Source: CAD feature listing. Evaluate the final solid. Frame: model axes, mm. A direction names the side the tool comes from. Round coordinates to 2 decimals unless told otherwise and drop trailing zeros. Loops run counter-clockwise (first coordinate to the right, second up) from the corner with the lowest first, then second, coordinate; pieces in that order, holes last. Notation, with made-up numbers: M 62,-30 L 111,-30 A20 ccw 111,-10 Z; hole C 21,38 d9. An arc over 180 degrees is marked long. Write each question's results on one line, items separated by ' | '. Start each with the question number.
1. Section B-B on z = -5. Output: boundary loops of the cut face in (x, y), and give its area (3 significant figures).
2. Draft query along Z for faces 1 (the flat face through (20, 3, -30)), 2 (the flat face through (0, 3, -15)), 3 (the cylindrical face through (36.464, 3.042, -4.675)). Return one class per face: released by +Z, released by -Z, zero draft, split by the parting line, or undercut.
3. Section A-A on x = 16. Output: boundary loops of the cut face in (y, z).
4. Set-up query: faces 4 (the flat face through (15.5, 5, -15)), 5 (the flat face through (25.5, 5.4, -15)), 6 (the flat face through (11.22, 1.53, -14.87)). Return all of +Z, -Z, +X, -X, +Y, -Y with unobstructed straight access to the full face (end or side cutting, diameter ignored); none if empty.
5. Contact query for flat-ended pins moving along their axis: pin 1 Ø5 at (x, z) = (35, -25) entering from +Y; pin 2 Ø2 at (x, z) = (16, -24) entering from +Y. Output: stop coordinate, or through.
6. Ray query, line 1 (X direction, y = 3.85, z = -25); line 2 (Z direction, x = 21, y = 5.75); line 3 (X direction, y = 1.55, z = -25). Return the intervals inside material, ascending.
7. Section C-C on x = 35. Output: boundary loops of the cut face in (y, z).
8. Section D-D on y = 0.5. Output: boundary loops of the cut face in (x, z).
from build123d import *
from OCP.BRepFilletAPI import BRepFilletAPI_MakeChamfer

# Parameters (mm, degrees)
SKETCH1_W           = 40
SKETCH1_H           = 30
BOSS_EXTRUDE1_DEPTH = 6
SKETCH2_R           = 1.5
CUT_EXTRUDE1_DEPTH  = 6
FILLET1_R           = 4
SKETCH3_W           = 21
SKETCH3_H           = 21
CUT_EXTRUDE2_DEPTH  = 4
SKETCH6_W           = 9
SKETCH6_H           = 5
CUT_EXTRUDE3_DEPTH  = 2
SKETCH7_W           = 11
SKETCH7_H           = 7
SKETCH7_W_2         = 9
SKETCH7_H_2         = 5
BOSS_EXTRUDE2_DEPTH = 4
CHAMFER1_SIZE       = 4
CHAMFER1_SIZE2      = 6.92820323
CHAMFER2_SIZE       = 2.886751346
CHAMFER2_SIZE_2     = 5


with BuildPart() as part:
    # Sketch1 → Boss-Extrude1 (new body)
    with BuildSketch(Plane(origin=(0, 0, 0), x_dir=(1, 0, 0), z_dir=(0, 1, 0))):
        with Locations((20, 15)):
            Rectangle(SKETCH1_W, SKETCH1_H)
    extrude(amount=BOSS_EXTRUDE1_DEPTH)

    # Sketch2 → Cut-Extrude1 (cut)
    with BuildSketch(Plane(origin=(0, 6, 0), x_dir=(1, 0, 0), z_dir=(0, 1, 0))):
        with Locations(Location((5, 5, 0), (0, 0, 270))):
            Circle(SKETCH2_R)
        with Locations(Location((5, 25, 0), (0, 0, 90))):
            Circle(SKETCH2_R)
        with Locations(Location((35, 5, 0), (0, 0, 90))):
            Circle(SKETCH2_R)
        with Locations(Location((35, 25, 0), (0, 0, 270))):
            Circle(SKETCH2_R)
    extrude(amount=-CUT_EXTRUDE1_DEPTH, mode=Mode.SUBTRACT)

    # Fillet1
    fillet1_edges = [part.edges().sort_by_distance(p)[0] for p in [
        (0, 3, -30),
        (40, 3, -30),
        (40, 3, 0),
        (0, 3, 0),
    ]]
    fillet(fillet1_edges, radius=FILLET1_R)

    # Sketch3 → Cut-Extrude2 (cut)
    with BuildSketch(Plane(origin=(0, 6, 0), x_dir=(1, 0, 0), z_dir=(0, 1, 0))):
        with Locations((20, 15)):
            Rectangle(SKETCH3_W, SKETCH3_H)
    extrude(amount=-CUT_EXTRUDE2_DEPTH, mode=Mode.SUBTRACT)

    # Sketch6 → Cut-Extrude3 (cut)
    with BuildSketch(Plane(origin=(0, 2, 0), x_dir=(1, 0, 0), z_dir=(0, 1, 0))):
        with Locations((20, 15)):
            Rectangle(SKETCH6_W, SKETCH6_H)
    extrude(amount=-CUT_EXTRUDE3_DEPTH, mode=Mode.SUBTRACT)

    # Sketch7 → Boss-Extrude2 (add)
    with BuildSketch(Plane(origin=(0, 2, 0), x_dir=(1, 0, 0), z_dir=(0, 1, 0))):
        with Locations((20, 15)):
            Rectangle(SKETCH7_W, SKETCH7_H)
        with Locations((20, 15)):
            Rectangle(SKETCH7_W_2, SKETCH7_H_2, mode=Mode.SUBTRACT)
    extrude(amount=BOSS_EXTRUDE2_DEPTH)

    # Chamfer1: one chamfer whose edges measure the first distance from different faces: ONE call of the kernel's chamfer builder (chamfer() names one face for all edges)
    chamfer1_edges_1 = [part.edges().sort_by_distance(p)[0] for p in [
        (20, 0, -12.5),
    ]]
    chamfer1_side_1 = [part.faces().sort_by_distance(p)[0] for p in [
        (20, 3, -12.5),
    ]]
    chamfer1_edges_2 = [part.edges().sort_by_distance(p)[0] for p in [
        (24.5, 0, -15),
    ]]
    chamfer1_side_2 = [part.faces().sort_by_distance(p)[0] for p in [
        (24.5, 3, -15),
    ]]
    chamfer1_edges_3 = [part.edges().sort_by_distance(p)[0] for p in [
        (20, 0, -17.5),
    ]]
    chamfer1_side_3 = [part.faces().sort_by_distance(p)[0] for p in [
        (20, 3, -17.5),
    ]]
    chamfer1_edges_4 = [part.edges().sort_by_distance(p)[0] for p in [
        (15.5, 0, -15),
    ]]
    chamfer1_side_4 = [part.faces().sort_by_distance(p)[0] for p in [
        (15.5, 3, -15),
    ]]
    chamfer1 = BRepFilletAPI_MakeChamfer(part.part.solid().wrapped)
    for e in chamfer1_edges_1:
        chamfer1.Add(CHAMFER1_SIZE, CHAMFER1_SIZE2, e.wrapped, chamfer1_side_1[0].wrapped)  # the first distance lies on this face
    for e in chamfer1_edges_2:
        chamfer1.Add(CHAMFER1_SIZE, CHAMFER1_SIZE2, e.wrapped, chamfer1_side_2[0].wrapped)  # the first distance lies on this face
    for e in chamfer1_edges_3:
        chamfer1.Add(CHAMFER1_SIZE, CHAMFER1_SIZE2, e.wrapped, chamfer1_side_3[0].wrapped)  # the first distance lies on this face
    for e in chamfer1_edges_4:
        chamfer1.Add(CHAMFER1_SIZE, CHAMFER1_SIZE2, e.wrapped, chamfer1_side_4[0].wrapped)  # the first distance lies on this face
    add(Compound.cast(chamfer1.Shape()), mode=Mode.REPLACE)

    # Chamfer2
    # the kernel refuses this chamfer: 5, 2.886751346 mm, written as the material it adds along each edge
    with BuildSketch(Plane(origin=(14.5, 2, -31.435428773), x_dir=(0, 1, 0), z_dir=(0, 0, 1))) as chamfer2_piece_1_section:
        Polygon((CHAMFER2_SIZE, 0), (0, CHAMFER2_SIZE_2), (0, 0), align=None)
    chamfer2_piece_1 = extrude(amount=32.870857546, mode=Mode.PRIVATE)
    chamfer2_piece_1 = split(chamfer2_piece_1, bisect_by=Plane(origin=(13.883974596, 3.066987298, -31.435428773), z_dir=(-0.499999999999998, 0.8660254037844398, 0)), keep=Keep.TOP, mode=Mode.PRIVATE)
    chamfer2_piece_1 = split(chamfer2_piece_1, bisect_by=Plane(origin=(14.5, -1.436141454, -29.45157158), z_dir=(0, -0.8660254037844382, 0.500000000000001)), keep=Keep.TOP, mode=Mode.PRIVATE)
    chamfer2_piece_1 = split(chamfer2_piece_1, bisect_by=Plane(origin=(14.5, 12.797357386, -25.20157158), z_dir=(0, -0.8660254037844382, -0.500000000000001)), keep=Keep.TOP, mode=Mode.PRIVATE)
    with BuildSketch(Plane(origin=(14.5, 2, -31.435428773), x_dir=(0, 1, 0), z_dir=(0, 0, 1))) as chamfer2_piece_2_section:
        Polygon((CHAMFER2_SIZE, 0), (0, CHAMFER2_SIZE_2), (0, 0), align=None)
    chamfer2_piece_2 = extrude(amount=32.870857546, mode=Mode.PRIVATE)
    chamfer2_piece_2 = split(chamfer2_piece_2, bisect_by=Plane(origin=(14.5, -2.534217665, -28.817596984), z_dir=(0, 0.8660254037844398, -0.499999999999998)), keep=Keep.TOP, mode=Mode.PRIVATE)
    chamfer2_piece_2 = split(chamfer2_piece_2, bisect_by=Plane(origin=(14.5, -1.436141454, -29.45157158), z_dir=(0, -0.8660254037844382, 0.500000000000001)), keep=Keep.TOP, mode=Mode.PRIVATE)
    with BuildSketch(Plane(origin=(14.5, 2, -31.435428773), x_dir=(0, 1, 0), z_dir=(0, 0, 1))) as chamfer2_piece_3_section:
        Polygon((CHAMFER2_SIZE, 0), (0, CHAMFER2_SIZE_2), (0, 0), align=None)
    chamfer2_piece_3 = extrude(amount=32.870857546, mode=Mode.PRIVATE)
    chamfer2_piece_3 = split(chamfer2_piece_3, bisect_by=Plane(origin=(14.5, 11.699281175, -25.835546176), z_dir=(0, 0.8660254037844398, 0.49999999999999795)), keep=Keep.TOP, mode=Mode.PRIVATE)
    chamfer2_piece_3 = split(chamfer2_piece_3, bisect_by=Plane(origin=(14.5, 12.797357386, -25.20157158), z_dir=(0, -0.8660254037844382, -0.500000000000001)), keep=Keep.TOP, mode=Mode.PRIVATE)
    with BuildSketch(Plane(origin=(1.564571227, 2, -11.5), x_dir=(0, 1, 0), z_dir=(1, 0, 0))) as chamfer2_piece_4_section:
        Polygon((CHAMFER2_SIZE, 0), (0, CHAMFER2_SIZE_2), (0, 0), align=None)
    chamfer2_piece_4 = extrude(amount=36.870857546, mode=Mode.PRIVATE)
    chamfer2_piece_4 = split(chamfer2_piece_4, bisect_by=Plane(origin=(1.564571227, 3.066987298, -10.883974596), z_dir=(0, 0.8660254037844398, 0.49999999999999795)), keep=Keep.TOP, mode=Mode.PRIVATE)
    chamfer2_piece_4 = split(chamfer2_piece_4, bisect_by=Plane(origin=(8.79842842, 14.529408194, -11.5), z_dir=(-0.500000000000001, -0.8660254037844382, 0)), keep=Keep.TOP, mode=Mode.PRIVATE)
    chamfer2_piece_4 = split(chamfer2_piece_4, bisect_by=Plane(origin=(3.54842842, -1.436141454, -11.5), z_dir=(0.500000000000001, -0.8660254037844382, 0)), keep=Keep.TOP, mode=Mode.PRIVATE)
    with BuildSketch(Plane(origin=(1.564571227, 2, -11.5), x_dir=(0, 1, 0), z_dir=(1, 0, 0))) as chamfer2_piece_5_section:
        Polygon((CHAMFER2_SIZE, 0), (0, CHAMFER2_SIZE_2), (0, 0), align=None)
    chamfer2_piece_5 = extrude(amount=36.870857546, mode=Mode.PRIVATE)
    chamfer2_piece_5 = split(chamfer2_piece_5, bisect_by=Plane(origin=(4.182403016, -2.534217665, -11.5), z_dir=(-0.499999999999998, 0.8660254037844398, 0)), keep=Keep.TOP, mode=Mode.PRIVATE)
    chamfer2_piece_5 = split(chamfer2_piece_5, bisect_by=Plane(origin=(3.54842842, -1.436141454, -11.5), z_dir=(0.500000000000001, -0.8660254037844382, 0)), keep=Keep.TOP, mode=Mode.PRIVATE)
    with BuildSketch(Plane(origin=(25.5, 2, 1.435428773), x_dir=(0, 1, 0), z_dir=(0, 0, -1))) as chamfer2_piece_6_section:
        Polygon((CHAMFER2_SIZE, 0), (0, CHAMFER2_SIZE_2), (0, 0), align=None)
    chamfer2_piece_6 = extrude(amount=32.870857546, mode=Mode.PRIVATE)
    chamfer2_piece_6 = split(chamfer2_piece_6, bisect_by=Plane(origin=(26.116025404, 3.066987298, 1.435428773), z_dir=(0.499999999999998, 0.8660254037844398, 0)), keep=Keep.TOP, mode=Mode.PRIVATE)
    chamfer2_piece_6 = split(chamfer2_piece_6, bisect_by=Plane(origin=(25.5, 12.797357386, -4.79842842), z_dir=(0, -0.8660254037844382, 0.500000000000001)), keep=Keep.TOP, mode=Mode.PRIVATE)
    chamfer2_piece_6 = split(chamfer2_piece_6, bisect_by=Plane(origin=(25.5, -1.436141454, -0.54842842), z_dir=(0, -0.8660254037844382, -0.500000000000001)), keep=Keep.TOP, mode=Mode.PRIVATE)
    with BuildSketch(Plane(origin=(25.5, 2, 1.435428773), x_dir=(0, 1, 0), z_dir=(0, 0, -1))) as chamfer2_piece_7_section:
        Polygon((CHAMFER2_SIZE, 0), (0, CHAMFER2_SIZE_2), (0, 0), align=None)
    chamfer2_piece_7 = extrude(amount=32.870857546, mode=Mode.PRIVATE)
    chamfer2_piece_7 = split(chamfer2_piece_7, bisect_by=Plane(origin=(25.5, -2.534217665, -1.182403016), z_dir=(0, 0.8660254037844398, 0.49999999999999795)), keep=Keep.TOP, mode=Mode.PRIVATE)
    chamfer2_piece_7 = split(chamfer2_piece_7, bisect_by=Plane(origin=(25.5, -1.436141454, -0.54842842), z_dir=(0, -0.8660254037844382, -0.500000000000001)), keep=Keep.TOP, mode=Mode.PRIVATE)
    with BuildSketch(Plane(origin=(25.5, 2, 1.435428773), x_dir=(0, 1, 0), z_dir=(0, 0, -1))) as chamfer2_piece_8_section:
        Polygon((CHAMFER2_SIZE, 0), (0, CHAMFER2_SIZE_2), (0, 0), align=None)
    chamfer2_piece_8 = extrude(amount=32.870857546, mode=Mode.PRIVATE)
    chamfer2_piece_8 = split(chamfer2_piece_8, bisect_by=Plane(origin=(25.5, 11.699281175, -4.164453824), z_dir=(0, 0.8660254037844398, -0.499999999999998)), keep=Keep.TOP, mode=Mode.PRIVATE)
    chamfer2_piece_8 = split(chamfer2_piece_8, bisect_by=Plane(origin=(25.5, 12.797357386, -4.79842842), z_dir=(0, -0.8660254037844382, 0.500000000000001)), keep=Keep.TOP, mode=Mode.PRIVATE)
    with BuildSketch(Plane(origin=(38.435428773, 2, -18.5), x_dir=(0, 1, 0), z_dir=(-1, 0, 0))) as chamfer2_piece_9_section:
        Polygon((CHAMFER2_SIZE, 0), (0, CHAMFER2_SIZE_2), (0, 0), align=None)
    chamfer2_piece_9 = extrude(amount=36.870857546, mode=Mode.PRIVATE)
    chamfer2_piece_9 = split(chamfer2_piece_9, bisect_by=Plane(origin=(38.435428773, 3.066987298, -19.116025404), z_dir=(0, 0.8660254037844398, -0.499999999999998)), keep=Keep.TOP, mode=Mode.PRIVATE)
    chamfer2_piece_9 = split(chamfer2_piece_9, bisect_by=Plane(origin=(36.45157158, -1.436141454, -18.5), z_dir=(-0.500000000000001, -0.8660254037844382, 0)), keep=Keep.TOP, mode=Mode.PRIVATE)
    chamfer2_piece_9 = split(chamfer2_piece_9, bisect_by=Plane(origin=(31.20157158, 14.529408194, -18.5), z_dir=(0.500000000000001, -0.8660254037844382, 0)), keep=Keep.TOP, mode=Mode.PRIVATE)
    with BuildSketch(Plane(origin=(38.435428773, 2, -18.5), x_dir=(0, 1, 0), z_dir=(-1, 0, 0))) as chamfer2_piece_10_section:
        Polygon((CHAMFER2_SIZE, 0), (0, CHAMFER2_SIZE_2), (0, 0), align=None)
    chamfer2_piece_10 = extrude(amount=36.870857546, mode=Mode.PRIVATE)
    chamfer2_piece_10 = split(chamfer2_piece_10, bisect_by=Plane(origin=(31.835546176, 13.431331982, -18.5), z_dir=(-0.499999999999998, 0.8660254037844398, 0)), keep=Keep.TOP, mode=Mode.PRIVATE)
    chamfer2_piece_10 = split(chamfer2_piece_10, bisect_by=Plane(origin=(31.20157158, 14.529408194, -18.5), z_dir=(0.500000000000001, -0.8660254037844382, 0)), keep=Keep.TOP, mode=Mode.PRIVATE)
    add([chamfer2_piece_1, chamfer2_piece_2, chamfer2_piece_3, chamfer2_piece_4, chamfer2_piece_5, chamfer2_piece_6, chamfer2_piece_7, chamfer2_piece_8, chamfer2_piece_9, chamfer2_piece_10])


solid = part.part
Taken from the geometry:
1) outline: M 0,0 L 3.5,0 L 3.5,6 L 0,6 Z; M 6.5,0 L 33.5,0 L 33.5,6 L 30.5,6 L 30.5,2 L 9.5,2 L 9.5,6 L 6.5,6 Z; M 36.5,0 L 40,0 L 40,6 L 36.5,6 Z | area: 120 mm^2
2) face 1: released by -Z | face 2: zero draft | face 3: undercut
3) outline: M 0,-30 L 6,-30 L 6,-25.5 L 2,-25.5 L 2,-23.5 L 4.89,-18.5 L 6,-18.5 L 6,-17.5 L 4,-17.5 L 0,-24.43 Z; M 0,-5.57 L 4,-12.5 L 6,-12.5 L 6,-11.5 L 4.89,-11.5 L 2,-6.5 L 2,-4.5 L 6,-4.5 L 6,0 L 0,0 Z
4) face 4: +Y, -Y | face 5: +Y | face 6: -Y
5) pin 1: y = 6 | pin 2: y = 2.29
6) line 1: 0 to 3.5, 6.5 to 9.5, 30.5 to 33.5, 36.5 to 40 | line 2: -30 to -25.5, -18.5 to -17.5, -12.5 to -11.5, -4.5 to 0 | line 3: 0 to 3.5, 6.5 to 33.5, 36.5 to 40
7) outline: M 0,-30 L 6,-30 L 6,-26.5 L 0,-26.5 Z; M 0,-23.5 L 6,-23.5 L 6,-6.5 L 0,-6.5 Z; M 0,-3.5 L 6,-3.5 L 6,0 L 0,0 Z
8) outline: M 0,-26 A4 ccw 4,-30 L 36,-30 A4 ccw 40,-26 L 40,-4 A4 ccw 36,0 L 4,0 A4 ccw 0,-4 Z; hole C 5,-25 d3; hole C 5,-5 d3; hole M 9.44,-23.56 L 30.56,-23.56 L 30.56,-6.44 L 9.44,-6.44 Z; hole C 35,-25 d3; hole C 35,-5 d3
